Source: CAD feature listing. Evaluate the final solid. Frame: model axes, mm. Give positions to 0.01 mm unless a question says otherwise; leave off trailing zeros. Loops run counter-clockwise (first coordinate to the right, second up) from the corner with the lowest first, then second, coordinate; pieces in that order, holes last. Notation, with made-up numbers: (3, 36) - (42, 36) arc R20 ccw to (42, 49) - close; hole circle Ø5 at (65, 68.5). An arc over 180 degrees is marked (long way). Write each question's results on one line, items separated by ' | '. Start each with the question number.
(1) Pull-direction query (X, two-part tool) for faces 1 (the flat face through (0, 0, 4)), 2 (the conical face through (2.08, 1.96, -3.59)), 3 (the cylindrical face through (-1.222, 0.028, -1.594)); classes: pulls with the +X half, pulls with the -X half, needs draft (parallel to the pull), parting line crosses it, or undercut.
(2) Cut plane A-A on y = 1.4. Return the cut outline in (x, z).
(3) Material intervals for line 1 along X through (y, z) = (0.1, -0.75); line 2 along Z through (x, y) = (-1, 0.35); line 3 along X through (y, z) = (-0.3, 0.25), sorted ascending. Write a range as [from, to].
from build123d import *

# Parameters (mm, degrees)
EXTRUDE1_DEPTH = 2
SKETCH3_R      = 2.009
EXTRUDE2_DEPTH = 8.302967433


with BuildPart() as part:
    # Sketch1 → Extrude1 (new, symmetric)
    with BuildSketch(Plane(origin=(0, 0, 0), x_dir=(1, 0, 0), z_dir=(0, 1, 0))):
        Polygon((4.618802154, 0), (2.309401077, 4), (-2.309401077, 4), (-4.618802154, 0), (-2.309401077, -4), (2.309401077, -4), align=None)
    extrude(amount=EXTRUDE1_DEPTH, both=True)

    # Sketch2 → Cut-Revolve1 (revolve, cut)
    with BuildSketch(Plane(origin=(0, 0, 0), x_dir=(0, 0, -1), z_dir=(1, 0, 0))):
        Polygon((-4, 2), (-78.063973132, -17.845381789), (-78.063973132, 2), align=None)
    cut_revolve1 = revolve(axis=Axis((0, 0, 0), (0, 1, 0)), mode=Mode.SUBTRACT)

    # Mirror1: Cut-Revolve1 across plane
    add(cut_revolve1.mirror(Plane.ZX), mode=Mode.SUBTRACT)

    # Sketch3 → Extrude2 (cut, through all)
    with BuildSketch(Plane(origin=(0, 2, 0), x_dir=(1, 0, 0), z_dir=(0, 1, 0))):
        with Locations(Location((0, 0, 0), (0, 0, 270))):
            Circle(SKETCH3_R)
    extrude(amount=-EXTRUDE2_DEPTH, mode=Mode.SUBTRACT)


solid = part.part
Ans:
1) face 1: needs draft | face 2: pulls with the +X half | face 3: undercut
2) outline: (-4.62, 0) - (-2.31, -4) - (2.31, -4) - (4.62, 0) - (2.31, 4) - (-2.31, 4) - close; hole circle Ø4.02 at (0, 0)
3) line 1: [-4.19, -1.86], [1.86, 4.19] | line 2: [-4, -1.74], [1.74, 4] | line 3: [-4.47, -1.99], [1.99, 4.47]
